Answer from the drawing. Dimensions are ordinates in mm from the lowest x, y and z of the part. Coordinates: 2 decimals unless noted, no trailing zeros. Write each loop counter-clockwise with the first axis right and the second up, starting at its lowest first coordinate (ties: lowest second). Pieces come first, ordered by that corner, then holes. Notation, with made-up numbers: (65.25, 12.25) -> (120.25, 12.25) arc R29 cw to (120.25, 50.25) -> close; hole circle Ø8 at (-1, 41.25). An arc over 180 degrees is marked (long way). Return JSON: item names as keys, results as strings.
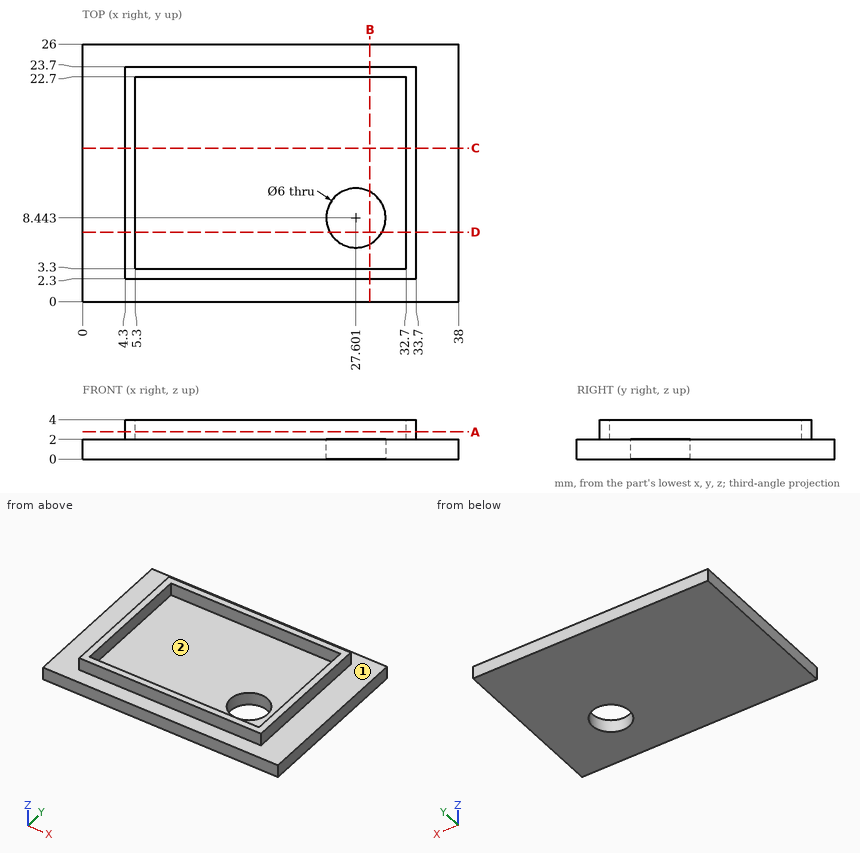
1. Flat-ended cylindrical pins translate along their axes: pin 1 Ø1.6 at (x, z) = (18.5, 2.5) entering from -Y; pin 2 Ø2 at (y, z) = (11, 3.5) entering from -X; pin 3 Ø1 at (y, z) = (14.5, 3) entering from +X; pin 4 Ø2 at (x, z) = (21, 3.5) entering from -Y. Find the tip coordinate at first contact, or state that the pin passes through.
Taken from the geometry:
{"pin 1": "stops at y = 0", "pin 2": "stops at x = 4.3", "pin 3": "stops at x = 33.7", "pin 4": "stops at y = 2.3"}
2. The part is cut by section D-D (y = 7). Determine the outline of the cut face in (x, z), then the cut area to 3 significant figures.
Taken from the geometry:
{"outline": "(0, 0) -> (24.97, 0) -> (24.97, 2) -> (5.3, 2) -> (5.3, 4) -> (4.3, 4) -> (4.3, 2) -> (0, 2) -> close; (30.23, 0) -> (38, 0) -> (38, 2) -> (33.7, 2) -> (33.7, 4) -> (32.7, 4) -> (32.7, 2) -> (30.23, 2) -> close", "area": "69.5 mm2"}
3. For a pull along Y with two mould halves and no side action, classify the marked faces 1 and 2 as +Y half, -Y half, draft (parallel to the pull), parting line (faces both ways), or undercut.
Taken from the geometry:
{"face 1": "draft", "face 2": "undercut"}
4. The part is cut by section B-B (x = 29). Determine the outline of the cut face in (y, z), then the cut area to 3 significant figures.
Taken from the geometry:
{"outline": "(0, 0) -> (5.79, 0) -> (5.79, 2) -> (3.3, 2) -> (3.3, 4) -> (2.3, 4) -> (2.3, 2) -> (0, 2) -> close; (11.1, 0) -> (26, 0) -> (26, 2) -> (23.7, 2) -> (23.7, 4) -> (22.7, 4) -> (22.7, 2) -> (11.1, 2) -> close", "area": "45.4 mm2"}
5. Consider L1, parallel to X at y = 10, z = 2.9; L2, parallel to Y at x = 21, z = 3.3; L3, parallel to Z at x = 6.5, y = 14.5. Determine where each line is inside the solid, lowest interval first.
Taken from the geometry:
{"L1": "x = 4.3 to 5.3, 32.7 to 33.7", "L2": "y = 2.3 to 3.3, 22.7 to 23.7", "L3": "z = 0 to 2"}
6. The part is cut by section A-A (z = 2.75). Determine the outline of the cut face in (x, y).
Taken from the geometry:
{"outline": "(4.3, 2.3) -> (33.7, 2.3) -> (33.7, 23.7) -> (4.3, 23.7) -> close; hole (5.3, 3.3) -> (32.7, 3.3) -> (32.7, 22.7) -> (5.3, 22.7) -> close"}
7. The part is cut by section C-C (y = 15.5). Determine the outline of the cut face in (x, z).
Taken from the geometry:
{"outline": "(0, 0) -> (38, 0) -> (38, 2) -> (33.7, 2) -> (33.7, 4) -> (32.7, 4) -> (32.7, 2) -> (5.3, 2) -> (5.3, 4) -> (4.3, 4) -> (4.3, 2) -> (0, 2) -> close"}
